Here's how the part is built. I have some questions about the finished solid (model axes, mm). A direction names the side the tool comes from. Round coordinates to 2 decimals unless told otherwise and drop trailing zeros. Write each loop counter-clockwise with the first axis right and the second up, starting at its lowest first coordinate (ties: lowest second). Pieces come first, ordered by that corner, then holes. Notation, with made-up numbers: M 65.25,-17.5 L 87.25,-17.5 A13 cw 87.25,-8.5 Z; hole C 55,-22.75 d10. An arc over 180 degrees is marked long. Use a Markdown table: item, result. Add a question column.
```python
from build123d import *

# Parameters (mm, degrees)
SKETCH2_R          = 4
CUT_EXTRUDE3_DEPTH = 36.503520952
CIRPATTERN1_COUNT  = 3


with BuildPart() as part:
    # Sketch1 → Revolve2 (revolve)
    with BuildSketch(Plane(origin=(0, 0, 0), x_dir=(0, 0, -1), z_dir=(1, 0, 0)), mode=Mode.PRIVATE) as revolve2_sk:
        Polygon((0, 0), (0, 14.975), (1, 15.975), (6, 15.975), (6, 16), (20, 16), (20, 18), (20.5, 18.5), (23, 18.5), (24, 17.5), (24, 14.077350269), (23, 13.5), (9, 13.5), (9, 13.75), (7, 13.75), (7, 11), (5, 11), (5, 1.5), (4.098709071, 0), align=None)
    revolve(revolve2_sk.sketch.rotate(Axis((0, 0, 0), (0, 0, -1)), 90), axis=Axis((0, 0, 0), (0, 0, -1)))

    # Sketch2 → Cut-Extrude3 (cut, through all)
    with BuildSketch(Plane(origin=(0, 0, 0), x_dir=(0, 0, -1), z_dir=(0, 1, 0))):
        with Locations((27.3, 0)):
            Circle(SKETCH2_R)
    cut_extrude3 = extrude(amount=CUT_EXTRUDE3_DEPTH, mode=Mode.SUBTRACT)

    # CirPattern1: Cut-Extrude3 ×3 about axis
    cirpattern1_axis = Axis((0, 0, -4.098709071), (0, 0, -1))
    for i in range(1, CIRPATTERN1_COUNT):
        add(cut_extrude3.rotate(cirpattern1_axis, i * 360 / CIRPATTERN1_COUNT), mode=Mode.SUBTRACT)


solid = part.part
```
Item 1: Imagine slicing it at B-B on z = -2.5. List the corners of the cut face in (x, y) for me (3 decimals).
Item 2: On a 3-axis mill with a long thin cutter (end or side, diameter ignored), from which of +Z, -Z, +X, -X, +Y, -Y can I reach the whole of each face in a straight line? I mean faces 4 (the face through (-2.93, 13.18, -15.9)), 5 (the face through (0, -15, -24)), 6 (the face through (0, 15.9, -23.3)). Say none if no direction works.
Item 3: Imagine slicing it at A-A on z = -9.5. List the corners of the cut face in (x, y) for me, plus the area to 3 significant figures.
Item 4: If we mould it in two halves opening along Y, with no side actions, what happens to faces 1 (the face through (12, 11, -20)), 2 (the face through (8.54, 16.41, -21.77)), 3 (the face through (-0.1, -11.3, -7))? For each: +Y half, -Y half, draft (parallel to the pull), parting line (faces both ways), or undercut.
Item 5: For pin 1 Ø6 at (x, y) = (1, 14) entering from +Z; pin 2 Ø5 at (y, z) = (4, -16) entering from -X; pin 3 Ø12 at (y, z) = (11, -9) entering from -X; pin 4 Ø1 at (y, z) = (-6.5, -16.5) entering from +X, each with a flat end and sliding along its axis, tell me the tip position at first contact or that it passes through.
Item 6: I need wall thicknesses on probe 1 along Y at (x, z) = (0, -12.5); probe 2 along Y at (x, z) = (0, -6.6); probe 3 along Z at (x, y) = (-8.5, -8.5). Which ranges of each line are inside material? Lowest first, please. Write a range as from..to.
The answers:
| question | item | result |
|---|---|---|
| 1 | outline | C 0,0 d31.95 |
| 2 | face 4 | -Z |
| 2 | face 5 | -Z, +X, -X, +Y, -Y |
| 2 | face 6 | -Z, +Y |
| 3 | outline | C 0,0 d32; hole C 0,0 d27 |
| 3 | area | 232 mm² |
| 4 | face 1 | draft |
| 4 | face 2 | parting line |
| 4 | face 3 | undercut |
| 5 | pin 1 | z = 0 |
| 5 | pin 2 | x = -15.93 |
| 5 | pin 3 | x = -15.2 |
| 5 | pin 4 | x = 14.83 |
| 6 | probe 1 | -16..-13.5, 13.5..16 |
| 6 | probe 2 | -16..-11, 11..16 |
| 6 | probe 3 | -7..0 |
